from build123d import *

# Parameters (mm, degrees)
BOSS_EXTRUDE4_DEPTH = 375
BOSS_EXTRUDE5_DEPTH = 7.5
CUT_EXTRUDE1_DEPTH  = 360
BOSS_EXTRUDE6_DEPTH = 32.5
LPATTERN1_COUNT     = 3
LPATTERN1_PITCH     = 160
LPATTERN1_COL_COUNT = 3
LPATTERN1_COL_PITCH = 160
SKETCH11_R          = 30
CUT_EXTRUDE2_DEPTH  = 1263.512529339
SKETCH12_R          = 60
SKETCH12_R_2        = 30
BOSS_EXTRUDE7_DEPTH = 32.5
SCALE_1_SCALE       = 0.1


with BuildPart() as part:
    # Sketch1 → Boss-Extrude4 (new, symmetric)
    with BuildSketch(Plane.XY):
        with BuildLine():
            Line((281.569977344, 264.00526259), (60.043258876, 0))
            Line((60.043258876, 0), (520.65961219, 0))
            ThreePointArc((520.65961219, 0), (564.907123778, 10.321921752), (600.02024832, 39.156845634))
            Line((600.02024832, 39.156845634), (730.44724808, 209.279019234))
            ThreePointArc((730.44724808, 209.279019234), (769.910899903, 304.081580706), (757.128519442, 405.97130652))
            Line((757.128519442, 405.97130652), (658.940406775, 648.676304078))
            ThreePointArc((658.940406775, 648.676304078), (613.16613298, 699.478789474), (545.447965883, 708.988074874))
            Line((545.447965883, 708.988074874), (493.401915404, 697.925345336))
            ThreePointArc((493.401915404, 697.925345336), (444.503904969, 671.828213907), (417.014937982, 623.698884104))
            Line((417.014937982, 623.698884104), (374.151637205, 447.112342165))
            ThreePointArc((374.151637205, 447.112342165), (338.436231819, 350.211710608), (281.569977344, 264.00526259))
        make_face()
    extrude(amount=BOSS_EXTRUDE4_DEPTH, both=True)

    # Sketch6 → Boss-Extrude5 (add, symmetric)
    with BuildSketch(Plane.XY.offset(140)):
        with BuildLine():
            Line((739.837232288, 602.21499348), (757.128519442, 405.97130652))
            Line((757.128519442, 405.97130652), (468.079651675, 688.843619215))
            ThreePointArc((468.079651675, 688.843619215), (438.909700759, 795.263431413), (549.226629435, 797.76097261))
            ThreePointArc((549.226629435, 797.76097261), (629.357941615, 754.030269249), (719.665800913, 740.692647386))
            ThreePointArc((719.665800913, 740.692647386), (801.063667795, 681.841548153), (739.837232288, 602.21499348))
        make_face()
    boss_extrude5 = extrude(amount=BOSS_EXTRUDE5_DEPTH, both=True)

    # Mirror2: Boss-Extrude5 across plane
    add(boss_extrude5.mirror(Plane.XY))

    # Sketch7 → Cut-Extrude1 (cut, symmetric)
    with BuildSketch(Plane.XY):
        with BuildLine():
            Line((60.410578327, 15), (329.990480538, 400))
            Line((329.990480538, 400), (404.359842809, 650))
            Line((404.359842809, 650), (608.375948196, 693.364961886))
            Line((608.375948196, 693.364961886), (698.639094975, 432.530508414))
            ThreePointArc((698.639094975, 432.530508414), (712.247197771, 292.899677108), (660.880251772, 162.349355884))
            Line((660.880251772, 162.349355884), (557.705122032, 15))
            Line((557.705122032, 15), (60.410578327, 15))
        make_face()
    extrude(amount=CUT_EXTRUDE1_DEPTH, both=True, mode=Mode.SUBTRACT)

    # Sketch10 → Boss-Extrude6 (add, symmetric)
    with BuildSketch(Plane.XY):
        Polygon((72.542939803, 30), (-77.392739815, 2.5), (-77.392739815, -2.5), (72.542939803, -30), (72.542939803, 0), align=None)
    boss_extrude6 = extrude(amount=BOSS_EXTRUDE6_DEPTH, both=True)

    # LPattern1: Boss-Extrude6 ×3
    with Locations(*[(0, 0, i * LPATTERN1_PITCH) for i in range(1, LPATTERN1_COUNT)]):
        add(boss_extrude6)

    # LPattern1 col: Boss-Extrude6 ×3
    with Locations(*[(0, 0, -i * LPATTERN1_COL_PITCH) for i in range(1, LPATTERN1_COL_COUNT)]):
        add(boss_extrude6)

    # Sketch11 → Cut-Extrude2 (cut, through all)
    with BuildSketch(Plane.XY.offset(147.5)):
        with Locations((495.043258876, 753.442101292)):
            Circle(SKETCH11_R)
        with Locations((731.794701004, 671.751442127)):
            Circle(SKETCH11_R)
    extrude(amount=-CUT_EXTRUDE2_DEPTH, mode=Mode.SUBTRACT)

    # Sketch12 → Boss-Extrude7 (add)
    with BuildSketch(Plane(origin=(0, 0, 132.5), x_dir=(-1, 0, 0), z_dir=(0, 0, -1))):
        with Locations((-731.794701004, 671.751442127)):
            Circle(SKETCH12_R)
        with Locations(Location((-731.794701004, 671.751442127, 0), (0, 0, 180))):
            Circle(SKETCH12_R_2, mode=Mode.SUBTRACT)
    boss_extrude7 = extrude(amount=BOSS_EXTRUDE7_DEPTH)

    # Mirror3: Boss-Extrude7 across plane
    add(boss_extrude7.mirror(Plane.XY))


with BuildPart() as part_1:
    # Scale 1: scaled about (560.789704791, 327.896781874, 0)
    add(part.part.scale(SCALE_1_SCALE).moved(Location((504.710734312, 295.107103687, 0))))


solid = part_1.part
Check sheet for the modelled part. Datum: model origin and axes. Units: mm. A direction names the side the tool comes from. Give positions to 0.01 mm unless a question says otherwise; leave off trailing zeros. Write each loop counter-clockwise with the first axis right and the second up, starting at its lowest first coordinate (ties: lowest second). Pieces come first, ordered by that corner, then holes. Notation, with made-up numbers: (42, -9) -> (98, -9) arc R17 ccw to (98, 16) -> close; hole circle Ø4 at (41, 5). An arc over 180 degrees is marked (long way). Write item = value, one per line.
Item 1: Gauge pin test, flat ends, axial feed: pin 1 (5 mm diameter, centred on y = 332, z = 17, fed in from +X); pin 2 (0.9 mm diameter, centred on y = 293.5, z = 33.5, fed in from +X) (3 decimals); pin 3 (1.7 mm diameter, centred on y = 297, z = 33.5, fed in from +X). Record the tip position at first contact, or that the pin passes through.
Output:
pin_1 = 581.84
pin_2 = 511.965
pin_3 = 563.66
Item 2: Sectioned sample at C-C on x = 509. Record the boundary of the cut face in (y, z).
Output:
outline = (292.65, -35.25) -> (297.56, -35.25) -> (297.56, -28.75) -> (292.65, -28.75) -> close; (292.65, -19.25) -> (297.56, -19.25) -> (297.56, -12.75) -> (292.65, -12.75) -> close; (292.65, -3.25) -> (297.56, -3.25) -> (297.56, 3.25) -> (292.65, 3.25) -> close; (292.65, 12.75) -> (297.56, 12.75) -> (297.56, 19.25) -> (292.65, 19.25) -> close; (292.65, 28.75) -> (297.56, 28.75) -> (297.56, 35.25) -> (292.65, 35.25) -> close
Item 3: Sectioned sample at D-D on x = 563. Record the boundary of the cut face in (y, z), and give its area (3 significant figures).
Output:
outline = (297.28, -37.5) -> (366.08, -37.5) -> (366.08, -14.75) -> (372.59, -14.75) -> (372.59, -13.25) -> (366.08, -13.25) -> (366.08, 13.25) -> (372.59, 13.25) -> (372.59, 14.75) -> (366.08, 14.75) -> (366.08, 37.5) -> (297.28, 37.5) -> close; hole (300.2, -36) -> (363.9, -36) -> (363.9, 36) -> (300.2, 36) -> close
area = 594 mm^2
Item 4: Sectioned sample at A-A on z = -21.5. Record the boundary of the cut face in (x, y) (3 decimals), and give its area (3 significant figures).
Output:
outline = (510.715, 295.107) -> (556.777, 295.107) arc R10 ccw to (564.713, 299.023) -> (577.755, 316.035) arc R20 ccw to (580.424, 335.704) -> (570.605, 359.975) arc R10 ccw to (559.256, 366.006) -> (554.051, 364.9) arc R10 ccw to (547.816, 360.674) -> (565.548, 364.444) -> (574.575, 338.36) arc R30 cw to (570.799, 311.342) -> (560.481, 296.607) -> (511.974, 296.607) -> close
area = 395 mm^2
Item 5: Tool access check on faces 4 (the flat face through (575.583, 347.67, -25.966)), 5 (the cylindrical face through (574.66, 367.34, 11.65)), 6 (the flat face through (556.69, 365.46, 26.28)), 7 (the flat face through (504.57, 296.75, -15.95)), 8 (the flat face through (556.69, 365.46, -25.97)). Record the directions out of +Z, -Z, +X, -X, +Y, -Y that give a thin tool (end or side, any length) a straight path to the whole face; none if there is none.
Output:
face_4 = -Z, +X, +Y
face_5 = none
face_6 = +Z, -X, +Y
face_7 = +Z, -Z, -X, +Y
face_8 = -Z, -X, +Y
Item 6: Scan lines: probe 1 along Z at (x, y) = (575, 367); probe 2 along Z at (x, y) = (563, 332.5); probe 3 along Y at (x, z) = (518, 18). Record each from-to range of solid material in increasing order. Write a range as from..to.
Output:
probe_1 = -14.75..-10, 10..14.75
probe_2 = -37.5..-36, 36..37.5
probe_3 = 295.11..296.61
Item 7: Sectioned sample at B-B on y = 323.5. Record the boundary of the cut face in (x, z).
Output:
outline = (534.45, -37.5) -> (581.32, -37.5) -> (581.32, 37.5) -> (534.45, 37.5) -> (534.45, 36) -> (575.8, 36) -> (575.8, -36) -> (534.45, -36) -> close
Item 8: Release check for a two-part mould opening along Z. For faces 1 (the flat face through (554, 323, -37.5)), 2 (the flat face through (556.558, 362.533, 0.504)), 3 (the flat face through (504.57, 296.75, 0.05)) record: +Z half, -Z half, draft (parallel to the pull), parting line (faces both ways), or undercut.
Output:
face_1 = -Z half
face_2 = undercut
face_3 = draft
